Can you work these out from the model? Positions are in its coordinate system, mm. Round coordinates to 2 decimals unless told otherwise and drop trailing zeros. Order: outer loops, then holes, each group sorted by start corner. A loop starts at its lowest first (then second) coordinate and runs counter-clockwise, first axis right, second up.
Autodesk Inventor part; units mm, degrees
ref_plane "YZ Plane" through (0, 0, 0) normal (1, 0, 0) x (0, 1, 0)
ref_plane "XZ Plane" through (0, 0, 0) normal (0, 1, 0) x (-1, 0, 0)
ref_plane "XY Plane" through (0, 0, 0) normal (0, 0, 1) x (1, 0, 0)
sketch "Sketch1" plane through (0, 0, 0) normal (0, 0, 1) x (1, 0, 0)
  point P0 (0, 0)
sketch "Sketch2" plane through (0, 0, 0) normal (0, 0, 1) x (1, 0, 0)
  line L0 (0, 0) -> (238.125, 0)
  line L1 (238.125, 0) -> (238.125, 266.7)
  line L2 (238.125, 266.7) -> (0, 266.7)
  line L3 (0, 266.7) -> (0, 0)
  line L4 (82.55, 0) -> (107.95, 0)
  line L5 (107.95, 0) -> (107.95, 31.75)
  line L6 (107.95, 31.75) -> (82.55, 31.75)
  line L7 (82.55, 31.75) -> (82.55, 0)
  line L8 (152.4, 0) -> (177.8, 0)
  line L9 (177.8, 0) -> (177.8, 31.75)
  line L10 (177.8, 31.75) -> (152.4, 31.75)
  line L11 (152.4, 31.75) -> (152.4, 0)
  line L12 (130.175, 266.7) -> (130.175, 0)
  dimension "Width" = 238.125
  dimension "d1" = 266.7
  dimension "d2" = 130.175
  dimension "d3" = 22.225
  dimension "d4" = 25.4
  dimension "d5" = 22.225
  dimension "d6" = 25.4
  dimension "d7" = 31.75
extrude "Extrusion1" add sketch "Sketch2" along normal mid plane 12.7 contours L3 L2 L12 L0 L5 L6 L7 | L2 L1 L0 L9 L10 L11 L12
equation "\"d1\" = Height + Thick"
equation "\"d8\" = Thick"
properties part number "SideWall"
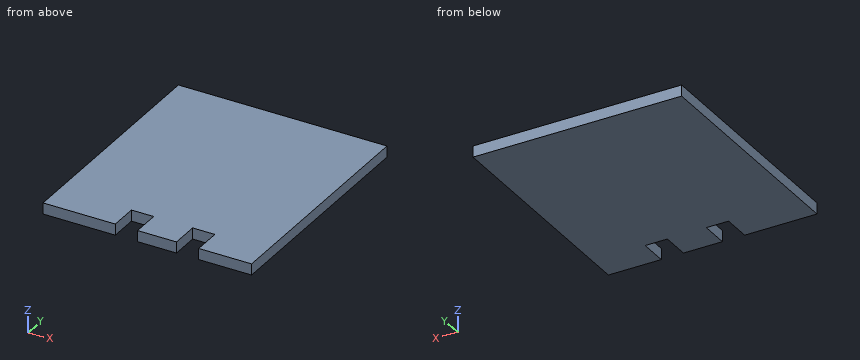
(1) I want a section at C-C, the plane x = 173. List the corners of the cut face in (y, z) for me, plus the area to 3 significant figures.
(2) I want a section at B-B, the plane z = -2. List the corners of the cut face in (x, y) for me (3 decimals).
(3) Please list where these lines run through material, in increasing order: probe 1 along X at (y, z) = (25, 1.25) (3 decimals); probe 2 along Y at (x, z) = (163, 1.5).
(4) I want a section at A-A, the plane y = 17.5. List the corners of the cut face in (x, z) for me (3 decimals), plus the area to 3 significant figures.
Ans:
1. outline: (31.75, -6.35) - (266.7, -6.35) - (266.7, 6.35) - (31.75, 6.35) - close
1. area: 2,980 mm2
2. outline: (0, 0) - (82.55, 0) - (82.55, 31.75) - (107.95, 31.75) - (107.95, 0) - (152.4, 0) - (152.4, 31.75) - (177.8, 31.75) - (177.8, 0) - (238.125, 0) - (238.125, 266.7) - (0, 266.7) - close
3. probe 1: x = 0 to 82.55, 107.95 to 152.4, 177.8 to 238.125
3. probe 2: y = 31.75 to 266.7
4. outline: (0, -6.35) - (82.55, -6.35) - (82.55, 6.35) - (0, 6.35) - close; (107.95, -6.35) - (152.4, -6.35) - (152.4, 6.35) - (107.95, 6.35) - close; (177.8, -6.35) - (238.125, -6.35) - (238.125, 6.35) - (177.8, 6.35) - close
4. area: 2,380 mm2
